Source: CAD feature listing. Evaluate the final solid. Frame: model axes, mm. A direction names the side the tool comes from. Coordinates: 2 decimals unless noted, no trailing zeros. Order: outer loops, then holes, each group sorted by start corner. A loop starts at its lowest first (then second) coordinate and runs counter-clockwise, first axis right, second up.
```python
from build123d import *

# Parameters (mm, degrees)
SKETCH1_R           = 22.225
SKETCH1_R_2         = 15.875
BOSS_EXTRUDE1_DEPTH = 3.175
SKETCH1_4_R         = 15.875
SKETCH1_4_R_2       = 10.4
BOSS_EXTRUDE2_DEPTH = 9.525
BOSS_EXTRUDE3_START = -6.35
SKETCH2_R           = 10.4
SKETCH2_R_2         = 3.05
BOSS_EXTRUDE3_DEPTH = 6.35
CHAMFER2_SIZE       = 3


with BuildPart() as part:
    # Sketch1 → Boss-Extrude1 (new body)
    with BuildSketch(Plane(origin=(0, 0, 0), x_dir=(1, 0, 0), z_dir=(0, 1, 0))):
        with Locations(Location((0, 0, 0), (0, 0, 270))):
            Circle(SKETCH1_R)
        with Locations(Location((0, 0, 0), (0, 0, 270))):
            Circle(SKETCH1_R_2, mode=Mode.SUBTRACT)
    extrude(amount=BOSS_EXTRUDE1_DEPTH)

    # Sketch1_4 → Boss-Extrude2 (add)
    with BuildSketch(Plane(origin=(0, 0, 0), x_dir=(1, 0, 0), z_dir=(0, 1, 0))):
        with Locations(Location((0, 0, 0), (0, 0, 90))):
            Circle(SKETCH1_4_R)
        with Locations(Location((0, 0, 0), (0, 0, 90))):
            Circle(SKETCH1_4_R_2, mode=Mode.SUBTRACT)
    extrude(amount=BOSS_EXTRUDE2_DEPTH)

    # Sketch2 → Boss-Extrude3 (add)
    with BuildSketch(Plane(origin=(0, 9.525, 0), x_dir=(1, 0, 0), z_dir=(0, 1, 0)).offset(BOSS_EXTRUDE3_START)):
        with Locations(Location((0, 0, 0), (0, 0, 90))):
            Circle(SKETCH2_R)
        with Locations(Location((0, 0, 0), (0, 0, 270))):
            Circle(SKETCH2_R_2, mode=Mode.SUBTRACT)
    extrude(amount=BOSS_EXTRUDE3_DEPTH)

    # Chamfer2
    chamfer2_edges = [part.edges().sort_by_distance(p)[0] for p in [
        (0, 9.525, 15.875),
    ]]
    chamfer(chamfer2_edges, length=CHAMFER2_SIZE)


solid = part.part
```
Q1. Pin query (flat end, axial travel): P1, Ø1.5, axis at x = -5.5, y = 1, coming from the -Z side; P2, Ø7, axis at x = 0, z = 0, coming from the -Y side (3 decimals); P3, Ø1.5, axis at x = -10, y = 3.5, coming from the +Z side. Return the tip coordinate at first contact, or that it passes through.
Solutions:
P1: stops at z = -21.71
P2: stops at y = 3.175
P3: stops at z = 20.17
Q2. Section query A-A on x = 0. Output: boundary loops of the cut face in (y, z) (3 decimals), plus the area to 3 significant figures.
Solutions:
outline: (0, -22.225) - (3.175, -22.225) - (3.175, -15.875) - (6.525, -15.875) - (9.525, -12.875) - (9.525, -3.05) - (3.175, -3.05) - (3.175, -10.4) - (0, -10.4) - close; (0, 10.4) - (3.175, 10.4) - (3.175, 3.05) - (9.525, 3.05) - (9.525, 12.875) - (6.525, 15.875) - (3.175, 15.875) - (3.175, 22.225) - (0, 22.225) - close
area: 229 mm2
Q3. Section query C-C on y = 5.25. Output: boundary loops of the cut face in (x, z) (3 decimals).
Solutions:
outline: circle Ø31.75 at (0, 0); hole circle Ø6.1 at (0, 0)
Q4. Pull-direction query (X, two-part tool) for faces 1 (the cylindrical face through (-1.856, 6.306, -2.42)), 2 (the cylindrical face through (15.497, 4.827, 3.441)), 3 (the flat face through (-5, 0, 10)); classes: pulls with the +X half, pulls with the -X half, needs draft (parallel to the pull), parting line crosses it, or undercut.
Solutions:
face 1: undercut
face 2: parting line crosses it
face 3: needs draft
Q5. Section query D-D on y = 8.5. Output: boundary loops of the cut face in (x, z).
Solutions:
outline: circle Ø27.8 at (0, 0); hole circle Ø6.1 at (0, 0)
Q6. Section query B-B on z = 0. Output: boundary loops of the cut face in (x, y) (3 decimals).
Solutions:
outline: (-22.225, 0) - (-10.4, 0) - (-10.4, 3.175) - (-3.05, 3.175) - (-3.05, 9.525) - (-12.875, 9.525) - (-15.875, 6.525) - (-15.875, 3.175) - (-22.225, 3.175) - close; (3.05, 3.175) - (10.4, 3.175) - (10.4, 0) - (22.225, 0) - (22.225, 3.175) - (15.875, 3.175) - (15.875, 6.525) - (12.875, 9.525) - (3.05, 9.525) - close
Q7. Material intervals for line 1 along X through (y, z) = (0.9, 0) (3 decimals); line 2 along Y through (x, z) = (11.5, -13.5) (3 decimals); line 3 along Y through (x, z) = (-0.5, 7.5) (3 decimals), sorted ascending.
Solutions:
line 1: x = -22.225 to -10.4, 10.4 to 22.225
line 2: y = 0 to 3.175
line 3: y = 3.175 to 9.525
Q8. Set-up query: faces 4 (the flat face through (2.2, 3.175, 2.5)), 5 (the cylindrical face through (18.74, 1.57, 11.95)), 6 (the flat face through (-15, 3.175, 10)). Return all of +Z, -Z, +X, -X, +Y, -Y with unobstructed straight access to the full face (end or side cutting, diameter ignored); none if empty.
Solutions:
face 4: -Y
face 5: +Y, -Y
face 6: +Y
